Work out the finished part from the listing and answer in its coordinate system (mm). A direction names the side the tool comes from. Coordinates: 2 decimals unless noted, no trailing zeros. Order: outer loops, then holes, each group sorted by start corner. A loop starts at its lowest first (then second) coordinate and runs counter-clockwise, first axis right, second up. Notation, with made-up numbers: M -35.5,-1 L -14.5,-1 A15 ccw -14.5,21 Z; hole C 86.5,72.5 d1. An arc over 180 degrees is marked long. Use a Markdown table: item, result.
from build123d import *

# Parameters (mm, degrees)
SKETCH5_R           = 2.1
BOSS_EXTRUDE1_DEPTH = 50


with BuildPart() as part:
    # Sketch5 → Boss-Extrude1 (new, symmetric)
    with BuildSketch(Plane(origin=(0, 0, 0), x_dir=(0, 0, -1), z_dir=(1, 0, 0))):
        with BuildLine():
            Line((-19.998019485, 4.9), (-18.198019485, 3.1))
            Line((-18.198019485, 3.1), (-18.198019485, 5.499339828))
            Line((-18.198019485, 5.499339828), (-16.558019485, 5.499339828))
            Line((-16.558019485, 5.499339828), (-13.9, 2.841320344))
            Line((-13.9, 2.841320344), (-13.9, -2.838679656))
            Line((-13.9, -2.838679656), (-16.558019485, -5.496699141))
            Line((-16.558019485, -5.496699141), (-18.198019485, -5.496699141))
            Line((-18.198019485, -5.496699141), (-18.198019485, -3.1))
            Line((-18.198019485, -3.1), (-19.998019485, -4.9))
            Line((-19.998019485, -4.9), (-19.998019485, -9))
            ThreePointArc((-19.998019485, -9), (-19.705126266, -9.707106781), (-18.998019485, -10))
            Line((-18.998019485, -10), (-14.9, -10))
            Line((-14.9, -10), (-13.1, -8.2))
            Line((-13.1, -8.2), (-15.5, -8.2))
            Line((-15.5, -8.2), (-15.5, -6.56))
            Line((-15.5, -6.56), (-12.84, -3.9))
            Line((-12.84, -3.9), (-7.16, -3.9))
            Line((-7.16, -3.9), (-4.5, -6.56))
            Line((-4.5, -6.56), (-4.5, -8.2))
            Line((-4.5, -8.2), (-6.9, -8.2))
            Line((-6.9, -8.2), (-5.1, -10))
            Line((-5.1, -10), (5.1, -10))
            Line((5.1, -10), (6.9, -8.2))
            Line((6.9, -8.2), (4.496038969, -8.2))
            Line((4.496038969, -8.2), (4.496038969, -6.56))
            Line((4.496038969, -6.56), (7.156038969, -3.9))
            Line((7.156038969, -3.9), (12.836038969, -3.9))
            Line((12.836038969, -3.9), (15.496038969, -6.56))
            Line((15.496038969, -6.56), (15.496038969, -8.2))
            Line((15.496038969, -8.2), (13.1, -8.2))
            Line((13.1, -8.2), (14.9, -10))
            Line((14.9, -10), (19.001980515, -10))
            ThreePointArc((19.001980515, -10), (19.709087297, -9.707106781), (20.001980515, -9))
            Line((20.001980515, -9), (20.001980515, -4.9))
            Line((20.001980515, -4.9), (18.201980515, -3.1))
            Line((18.201980515, -3.1), (18.201980515, -5.504621202))
            Line((18.201980515, -5.504621202), (16.561980515, -5.504621202))
            Line((16.561980515, -5.504621202), (13.9, -2.842640687))
            Line((13.9, -2.842640687), (13.9, 2.837359313))
            Line((13.9, 2.837359313), (16.561980515, 5.499339828))
            Line((16.561980515, 5.499339828), (18.201980515, 5.499339828))
            Line((18.201980515, 5.499339828), (18.201980515, 3.1))
            Line((18.201980515, 3.1), (20.001980515, 4.9))
            Line((20.001980515, 4.9), (20.001980515, 9))
            ThreePointArc((20.001980515, 9), (19.709087297, 9.707106781), (19.001980515, 10))
            Line((19.001980515, 10), (14.9, 10))
            Line((14.9, 10), (13.1, 8.2))
            Line((13.1, 8.2), (15.501320344, 8.2))
            Line((15.501320344, 8.2), (15.501320344, 6.56))
            Line((15.501320344, 6.56), (12.841320344, 3.9))
            Line((12.841320344, 3.9), (7.161320344, 3.9))
            Line((7.161320344, 3.9), (4.501320344, 6.56))
            Line((4.501320344, 6.56), (4.501320344, 8.2))
            Line((4.501320344, 8.2), (6.9, 8.2))
            Line((6.9, 8.2), (5.1, 10))
            Line((5.1, 10), (-5.1, 10))
            Line((-5.1, 10), (-6.9, 8.2))
            Line((-6.9, 8.2), (-4.501320344, 8.2))
            Line((-4.501320344, 8.2), (-4.501320344, 6.56))
            Line((-4.501320344, 6.56), (-7.161320344, 3.9))
            Line((-7.161320344, 3.9), (-12.841320344, 3.9))
            Line((-12.841320344, 3.9), (-15.501320344, 6.56))
            Line((-15.501320344, 6.56), (-15.501320344, 8.2))
            Line((-15.501320344, 8.2), (-13.1, 8.2))
            Line((-13.1, 8.2), (-14.9, 10))
            Line((-14.9, 10), (-18.998019485, 10))
            ThreePointArc((-18.998019485, 10), (-19.705126266, 9.707106781), (-19.998019485, 9))
            Line((-19.998019485, 9), (-19.998019485, 4.9))
        make_face()
        with Locations((-10, 0)):
            Circle(SKETCH5_R, mode=Mode.SUBTRACT)
        with Locations((10, 0)):
            Circle(SKETCH5_R, mode=Mode.SUBTRACT)
        Polygon((6.1, -2.84), (6.1, 2.84), (2.7, 6.24), (2.7, 8.2), (-2.7, 8.2), (-2.7, 6.24), (-6.1, 2.84), (-6.1, -2.84), (-2.7, -6.24), (-2.7, -8.2), (2.7, -8.2), (2.7, -6.24), align=None, mode=Mode.SUBTRACT)
        with BuildLine():
            Line((16.571320344, 8.2), (18.001980515, 8.2))
            ThreePointArc((18.001980515, 8.2), (18.143401872, 8.141421356), (18.201980515, 8))
            Line((18.201980515, 8), (18.201980515, 6.569339828))
            ThreePointArc((18.201980515, 6.569339828), (18.078517202, 6.384563922), (17.860559159, 6.427918472))
            Line((17.860559159, 6.427918472), (16.429898987, 7.858578644))
            ThreePointArc((16.429898987, 7.858578644), (16.386544437, 8.076536686), (16.571320344, 8.2))
        make_face(mode=Mode.SUBTRACT)
        with BuildLine():
            Line((16.571320344, -8.2), (18.001980515, -8.2))
            ThreePointArc((18.001980515, -8.2), (18.143401872, -8.141421356), (18.201980515, -8))
            Line((18.201980515, -8), (18.201980515, -6.569339828))
            ThreePointArc((18.201980515, -6.569339828), (18.078517202, -6.384563922), (17.860559159, -6.427918472))
            Line((17.860559159, -6.427918472), (16.429898987, -7.858578644))
            ThreePointArc((16.429898987, -7.858578644), (16.386544437, -8.076536686), (16.571320344, -8.2))
        make_face(mode=Mode.SUBTRACT)
        with BuildLine():
            Line((-17.860559159, 6.427918472), (-16.429898987, 7.858578644))
            ThreePointArc((-16.429898987, 7.858578644), (-16.386544437, 8.076536686), (-16.571320344, 8.2))
            Line((-16.571320344, 8.2), (-18.001980515, 8.2))
            ThreePointArc((-18.001980515, 8.2), (-18.143401872, 8.141421356), (-18.201980515, 8))
            Line((-18.201980515, 8), (-18.201980515, 6.569339828))
            ThreePointArc((-18.201980515, 6.569339828), (-18.078517202, 6.384563922), (-17.860559159, 6.427918472))
        make_face(mode=Mode.SUBTRACT)
        with BuildLine():
            Line((-16.571320344, -8.2), (-18.001980515, -8.2))
            ThreePointArc((-18.001980515, -8.2), (-18.143401872, -8.141421356), (-18.201980515, -8))
            Line((-18.201980515, -8), (-18.201980515, -6.569339828))
            ThreePointArc((-18.201980515, -6.569339828), (-18.078517202, -6.384563922), (-17.860559159, -6.427918472))
            Line((-17.860559159, -6.427918472), (-16.429898987, -7.858578644))
            ThreePointArc((-16.429898987, -7.858578644), (-16.386544437, -8.076536686), (-16.571320344, -8.2))
        make_face(mode=Mode.SUBTRACT)
    extrude(amount=BOSS_EXTRUDE1_DEPTH, both=True)


solid = part.part
(1) Given P1, Ø6, axis at x = 22, z = -11, coming from the -Y side; P2, Ø3, axis at x = 23, y = -1, coming from the +Z side; P3, Ø1.5, axis at x = 31, z = -13.5, coming from the -Y side; P4, Ø2.5, axis at x = -1.5, y = 4.5, coming from the -Z side, each flat-ended and moving along its own axis, determine where each tip first touches the part or whether it passes through.
Conclusion:
| item | result |
|---|---|
| P1 | y = -9.1 |
| P2 | z = 13.9 |
| P3 | y = -9.35 |
| P4 | z = -20 |
(2) A cutting plane is placed at B-B (y = 0). Determine the outline of the cut face in (x, z).
Conclusion:
| item | result |
|---|---|
| outline | M -50,-13.9 L 50,-13.9 L 50,-12.1 L -50,-12.1 Z; M -50,-7.9 L 50,-7.9 L 50,-6.1 L -50,-6.1 Z; M -50,6.1 L 50,6.1 L 50,7.9 L -50,7.9 Z; M -50,12.1 L 50,12.1 L 50,13.9 L -50,13.9 Z |
(3) Determine the mould class of faces 6 (the flat face through (1, -7, 19.998)), 7 (the flat face through (1, 8.2, 6)), 8 (the flat face through (1, -10, 0)), 9 (the flat face through (0.7, 5.25, -14.19)) for opening direction Y: pulls with the +Y half, pulls with the -Y half, needs draft (parallel to the pull), parting line crosses it, or undercut.
Conclusion:
| item | result |
|---|---|
| face 6 | needs draft |
| face 7 | undercut |
| face 8 | pulls with the -Y half |
| face 9 | undercut |
(4) A cutting plane is placed at A-A (z = 10). Determine the outline of the cut face in (x, y), then the cut area to 3 significant figures.
Conclusion:
| item | result |
|---|---|
| outline | M -50,-3.9 L 50,-3.9 L 50,-2.1 L -50,-2.1 Z; M -50,2.1 L 50,2.1 L 50,3.9 L -50,3.9 Z |
| area | 360 mm2 |
(5) Which of the six approach directions +Z, -Z, +X, -X, +Y, -Y give full straight-line access (tool end or side, diameter ignored) to faces 1 (the flat face through (0.7, 4, -19.1)), 2 (the flat face through (1, 0, 13.9)), 3 (the flat face through (0.7, -5.21, 5.85)), 4 (the flat face through (1, 7, 19.998)), 5 (the flat face through (1, -3.9, 10))?
Conclusion:
| item | result |
|---|---|
| face 1 | -Z, +X, -X |
| face 2 | +Z, +X, -X |
| face 3 | +X, -X |
| face 4 | +Z, +X, -X, +Y, -Y |
| face 5 | +X, -X, -Y |
(6) Straight lines are drawn through the part: L1, parallel to Z at x = 1.5, y = -9; L2, parallel to Y at x = 10, z = 10; L3, parallel to Y at x = 6.5, z = 16.5. For each, find the intervals that lie inside material, in ascending order.
Conclusion:
| item | result |
|---|---|
| L1 | -20 to -13.9, -6.1 to 6.1, 13.9 to 20 |
| L2 | -3.9 to -2.1, 2.1 to 3.9 |
| L3 | -10 to -8.19, -7.79 to -5.44, 5.44 to 7.79, 8.19 to 10 |
(7) A cutting plane is placed at C-C (x = 34.5). Give the number of separate pieces and of enclosed holes in the cut face, then the cut area to 3 significant figures.
Conclusion:
| item | result |
|---|---|
| separate pieces | 1 |
| enclosed holes | 7 |
| area | 285 mm2 |
